Input: dimensioned drawing with shaded views. Units: mm. Origin: part minimum x, y, z. Round coordinates to 2 decimals unless told otherwise and drop trailing zeros. Loops run counter-clockwise (first coordinate to the right, second up) from the corner with the lowest first, then second, coordinate; pieces in that order, holes last. Notation, with made-up numbers: (52, 70.5) - (86, 70.5) arc R13 cw to (86, 78.5) - close; hole circle Ø6 at (68.5, 55). An arc over 180 degrees is marked (long way). Use CSV: the item, a comma, the result in double quotes. Start each with the question number.
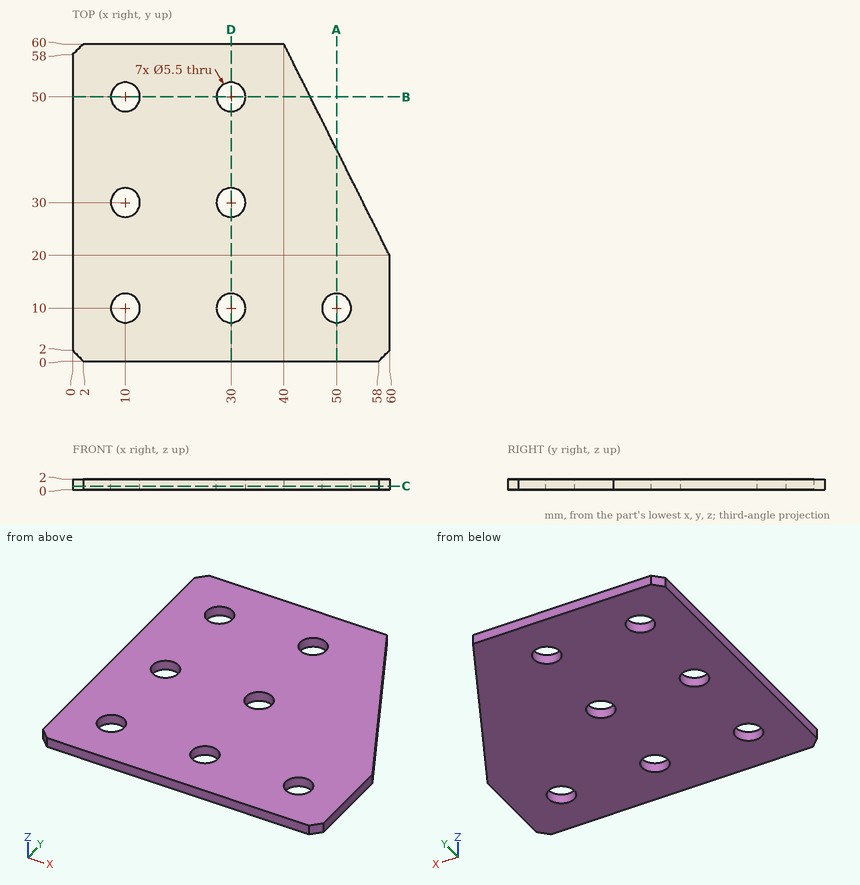
1. Section query B-B on y = 50. Return the cut outline in (x, z), and give its area (3 significant figures).
2. Section query D-D on x = 30. Return the cut outline in (y, z).
3. Section query A-A on x = 50. Return the cut outline in (y, z), and give its area (3 significant figures).
4. Section query C-C on z = 0.65. Return the cut outline in (x, y).
5. Line query: line 1 along Y through (x, z) = (10, 0.5); line 2 along X through (y, z) = (30, 0.8). Output: solid intervals per line, ascending.
Values:
1,outline,"(0, 0) - (7.25, 0) - (7.25, 2) - (0, 2) - close; (12.75, 0) - (27.25, 0) - (27.25, 2) - (12.75, 2) - close; (32.75, 0) - (45, 0) - (45, 2) - (32.75, 2) - close"
1,area,"68.0 mm^2"
2,outline,"(0, 0) - (7.25, 0) - (7.25, 2) - (0, 2) - close; (12.75, 0) - (27.25, 0) - (27.25, 2) - (12.75, 2) - close; (32.75, 0) - (47.25, 0) - (47.25, 2) - (32.75, 2) - close; (52.75, 0) - (60, 0) - (60, 2) - (52.75, 2) - close"
3,outline,"(0, 0) - (7.25, 0) - (7.25, 2) - (0, 2) - close; (12.75, 0) - (40, 0) - (40, 2) - (12.75, 2) - close"
3,area,"69.0 mm^2"
4,outline,"(0, 2) - (2, 0) - (58, 0) - (60, 2) - (60, 20) - (40, 60) - (2, 60) - (0, 58) - close; hole circle Ø5.5 at (10, 10); hole circle Ø5.5 at (10, 30); hole circle Ø5.5 at (10, 50); hole circle Ø5.5 at (30, 10); hole circle Ø5.5 at (30, 30); hole circle Ø5.5 at (30, 50); hole circle Ø5.5 at (50, 10)"
5,line 1,"y = 0 to 7.25, 12.75 to 27.25, 32.75 to 47.25, 52.75 to 60"
5,line 2,"x = 0 to 7.25, 12.75 to 27.25, 32.75 to 55"
